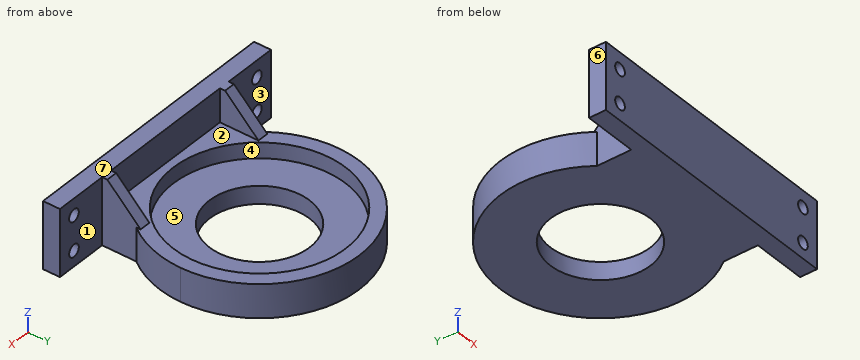
```python
from build123d import *

# Parameters (mm, degrees)
F0_W      = 24
F0_H      = 7.6146386564
F1_DEPTH  = 15
F2_R      = 38.75
F4_DEPTH  = 7
F5_DEPTH  = 15
F7_DEPTH  = 15
F8_SIZE   = 14.99999
F9_R      = 2.75
F10_DEPTH = 25
F11_R     = 22.5
F12_DEPTH = 25


# Not quite as in the source:
# - a fillet or chamfer is up to 0.001 mm smaller than in the source, because OpenCascade refuses the exact size


with BuildPart() as f1:
    # F0 (on Top) → F1 (new body)
    with BuildSketch(Plane.XY):
        with BuildLine():
            ThreePointArc((36, -27), (42.6907484123, -14.2302494708), (45, 0))
            ThreePointArc((45, 0), (-14.2302494708, 42.6907484123), (-36, -27))
            Line((-36, -27), (36, -27))
        make_face()
        with BuildLine():
            ThreePointArc((-15.1652218257, -42.3676297069), (-26.7116265289, -36.2144861648), (-36, -27))
            Line((-36, -27), (-36, -42.3676297069))
            Line((-36, -42.3676297069), (-15.1652218257, -42.3676297069))
        make_face()
        with BuildLine():
            Line((36, -27), (-36, -27))
            ThreePointArc((-36, -27), (-26.7116265289, -36.2144861648), (-15.1652218257, -42.3676297069))
            Line((-15.1652218257, -42.3676297069), (15.1652218257, -42.3676297069))
            ThreePointArc((15.1652218257, -42.3676297069), (26.7116265289, -36.2144861648), (36, -27))
        make_face()
        with BuildLine():
            Line((15.1652218257, -42.3676297069), (-15.1652218257, -42.3676297069))
            ThreePointArc((-15.1652218257, -42.3676297069), (0, -45), (15.1652218257, -42.3676297069))
        make_face()
        with Locations((-48, -46.174949035)):
            Rectangle(F0_W, F0_H)
        with BuildLine():
            ThreePointArc((15.1652218257, -42.3676297069), (0, -45), (-15.1652218257, -42.3676297069))
            Line((-15.1652218257, -42.3676297069), (-36, -42.3676297069))
            Line((-36, -42.3676297069), (-36, -49.9822683632))
            Line((-36, -49.9822683632), (36, -49.9822683632))
            Line((36, -49.9822683632), (36, -42.3676297069))
            Line((36, -42.3676297069), (15.1652218257, -42.3676297069))
        make_face()
        with Locations((48, -46.174949035)):
            Rectangle(F0_W, F0_H)
        with BuildLine():
            Line((36, -42.3676297069), (36, -27))
            ThreePointArc((36, -27), (26.7116265289, -36.2144861648), (15.1652218257, -42.3676297069))
            Line((15.1652218257, -42.3676297069), (36, -42.3676297069))
        make_face()
    extrude(amount=F1_DEPTH)

    # F2 (on face) → F4 (cut)
    with BuildSketch(Plane.XY.offset(15)):
        Circle(F2_R)
    extrude(amount=-F4_DEPTH, mode=Mode.SUBTRACT)

    # F3 (on face) → F5 (join)
    with BuildSketch(Plane.XY.offset(15)):
        Polygon((-36, -42.3676297069), (-60, -42.3676297069), (-60, -49.9822683632), (60, -49.9822683632), (60, -42.3676297069), (36, -42.3676297069), align=None)
    extrude(amount=F5_DEPTH)

    # F6 (on face) → F7 (join)
    with BuildSketch(Plane.XY.offset(15)):
        Polygon((-31, -25.031657964), (-36, -25.031657964), (-36, -27), (-36, -42.3676297069), (-31, -42.3676297069), align=None)
        Polygon((36, -42.3676297069), (36, -27), (36, -25.031657964), (31, -25.031657964), (31, -42.3676297069), align=None)
    extrude(amount=F7_DEPTH)

    # F8 (size 15 in the source; OpenCascade refuses exactly that, so slightly less here)
    f8_edges = [f1.edges().sort_by_distance(p)[0] for p in [
        (-33.5, -25.031658, 30),
        (33.5, -25.031658, 30),
    ]]
    chamfer(f8_edges, length=F8_SIZE)

    # F9 (on face) → F10 (cut)
    with BuildSketch(Plane(origin=(0, -42.3676297069, 0), x_dir=(-1, 0, 0), z_dir=(0, 1, 0))):
        with Locations((52, 7.5)):
            Circle(F9_R)
        with Locations((52, 22.5)):
            Circle(F9_R)
        with Locations((-52, 7)):
            Circle(F9_R)
        with Locations((-52, 22.5)):
            Circle(F9_R)
    extrude(amount=-F10_DEPTH, mode=Mode.SUBTRACT)

    # F11 (on face) → F12 (cut)
    with BuildSketch(Plane.XY.offset(8)):
        Circle(F11_R)
    extrude(amount=-F12_DEPTH, mode=Mode.SUBTRACT)


solid = f1.part
```
Geometry check sheet. Reference: the model listing, model coordinates, mm. Face numbers are marked on the shaded views. A direction names the side the tool comes from. Coordinates: 2 decimals unless noted, no trailing zeros. Loops run counter-clockwise (first coordinate to the right, second up) from the corner with the lowest first, then second, coordinate; pieces in that order, holes last.
Item 1: Sectioned sample at C-C, the plane y = 2. Record the boundary of the cut face in (x, z).
Item 2: Access from +Z, -Z, +X, -X, +Y, -Y to the whole of each face (thin tool, end or side, straight path). Record for the marked faces 1, 2, 3 and 4.
Item 3: Thickness scan on line 1 (Z direction, x = 52, y = -44); line 2 (Y direction, x = 0, z = 12); line 3 (Z direction, x = -52, y = -46). Record the ranges inside material, lowest first.
Item 4: Go/stop test with flat-tipped pins: pin 1 Ø14 at (y, z) = (-29.5, 8.5) entering from -X; pin 2 Ø7 at (x, z) = (51, 18) entering from +Y; pin 3 Ø5 at (y, z) = (8, 6.5) entering from -X. Record where each tip stops, or that it passes through.
Item 5: Sectioned sample at B-B, the plane x = 0. Record the boundary of the cut face in (y, z).
Item 6: Sectioned sample at A-A, the plane x = 52. Record the boundary of the cut face in (y, z), then the cut area to 3 significant figures.
Item 7: Sectioned sample at D-D, the plane z = 22.5. Record the boundary of the cut face in (x, y).
Item 8: Release check for a two-part mould opening along X. For the marked faces 5, 6 and 7 record: released by +X, released by -X, zero draft, split by the parting line, or undercut.
Check result:
1. outline: (-44.96, 0) - (-22.41, 0) - (-22.41, 8) - (-38.7, 8) - (-38.7, 15) - (-44.96, 15) - close; (22.41, 0) - (44.96, 0) - (44.96, 15) - (38.7, 15) - (38.7, 8) - (22.41, 8) - close
2. face 1: +Z, -Z, +X
2. face 2: +Z, +Y
2. face 3: +Z, -Z, -X
2. face 4: +Z
3. line 1: z = 0 to 4.25, 9.75 to 19.75, 25.25 to 30
3. line 2: y = -49.98 to -38.75, 38.75 to 45
3. line 3: z = 0 to 4.75, 10.25 to 19.75, 25.25 to 30
4. pin 1: stops at x = -38.97
4. pin 2: stops at y = -42.37
4. pin 3: stops at x = -44.66
5. outline: (-49.98, 0) - (-22.5, 0) - (-22.5, 8) - (-38.75, 8) - (-38.75, 15) - (-42.37, 15) - (-42.37, 30) - (-49.98, 30) - close; (22.5, 0) - (45, 0) - (45, 15) - (38.75, 15) - (38.75, 8) - (22.5, 8) - close
6. outline: (-49.98, 0) - (-42.37, 0) - (-42.37, 4.25) - (-49.98, 4.25) - close; (-49.98, 9.75) - (-42.37, 9.75) - (-42.37, 19.75) - (-49.98, 19.75) - close; (-49.98, 25.25) - (-42.37, 25.25) - (-42.37, 30) - (-49.98, 30) - close
6. area: 145 mm2
7. outline: (-60, -49.98) - (-54.75, -49.98) - (-54.75, -42.37) - (-60, -42.37) - close; (-49.25, -49.98) - (49.25, -49.98) - (49.25, -42.37) - (36, -42.37) - (36, -32.53) - (31, -32.53) - (31, -42.37) - (-31, -42.37) - (-31, -32.53) - (-36, -32.53) - (-36, -42.37) - (-49.25, -42.37) - close; (54.75, -49.98) - (60, -49.98) - (60, -42.37) - (54.75, -42.37) - close
8. face 5: undercut
8. face 6: released by -X
8. face 7: zero draft
